```python
from build123d import *

# Parameters (mm, degrees)
F0_R     = 19.05
F1_DEPTH = 31.75
F2_R     = 5.5626
F3_DEPTH = 20.6502
F4_DEPTH = 57.151
F6_DEPTH = 4.7625


with BuildPart() as f1:
    # F0 (on Front) → F1 (new body, symmetric)
    with BuildSketch(Plane.XZ):
        with BuildLine():
            Line((50.8, 28.575), (0, 28.575))
            ThreePointArc((0, 28.575), (-15.0603473566, -24.2840804335), (25.5976683508, 12.7))
            Line((25.5976683508, 12.7), (50.8, 12.7))
            Line((50.8, 12.7), (50.8, 28.575))
        make_face()
        Circle(F0_R, mode=Mode.SUBTRACT)
    extrude(amount=F1_DEPTH, both=True)

    # F2 (on face) → F3 (join)
    with BuildSketch(Plane(origin=(0, 0, 12.7), x_dir=(1, 0, 0), z_dir=(0, 0, -1))):
        with BuildLine():
            Line((50.8, 24.6126), (50.8, 31.75))
            ThreePointArc((50.8, 31.75), (41.8197438789, 28.0302561211), (38.1, 19.05))
            Line((38.1, 19.05), (38.1, -19.05))
            ThreePointArc((38.1, -19.05), (41.8197438789, -28.0302561211), (50.8, -31.75))
            Line((50.8, -31.75), (50.8, -24.6126))
            ThreePointArc((50.8, -24.6126), (45.2374, -19.05), (50.8, -13.4874))
            Line((50.8, -13.4874), (50.8, 13.4874))
            ThreePointArc((50.8, 13.4874), (45.2374, 19.05), (50.8, 24.6126))
        make_face()
        with BuildLine():
            Line((90.4493554441, 11.0277214642), (57.0991554441, 30.0777214642))
            ThreePointArc((57.0991554441, 30.0777214642), (54.0586759125, 31.3248128824), (50.8, 31.75))
            Line((50.8, 31.75), (50.8, 24.6126))
            ThreePointArc((50.8, 24.6126), (54.733352181, 22.983352181), (56.3626, 19.05))
            ThreePointArc((56.3626, 19.05), (54.733352181, 15.116647819), (50.8, 13.4874))
            Line((50.8, 13.4874), (50.8, -13.4874))
            ThreePointArc((50.8, -13.4874), (54.733352181, -15.116647819), (56.3626, -19.05))
            ThreePointArc((56.3626, -19.05), (54.733352181, -22.983352181), (50.8, -24.6126))
            Line((50.8, -24.6126), (50.8, -31.75))
            ThreePointArc((50.8, -31.75), (54.0586759125, -31.3248128824), (57.0991554441, -30.0777214642))
            Line((57.0991554441, -30.0777214642), (90.4493554441, -11.0277214642))
            ThreePointArc((90.4493554441, -11.0277214642), (96.8502, 0), (90.4493554441, 11.0277214642))
        make_face()
        with Locations((84.1502, 0)):
            Circle(F2_R, mode=Mode.SUBTRACT)
    extrude(amount=-F3_DEPTH)

    # F4 (cut, through all): faces of the model
    f4_faces = [f1.faces().sort_by_distance(p)[0] for p in [
        (48.4391592362, 19.05, 28.575),
        (48.4391592362, -19.05, 28.575),
    ]]
    extrude(f4_faces, amount=-F4_DEPTH, mode=Mode.SUBTRACT)

    # F5 (on Front) → F6 (join, symmetric)
    with BuildSketch(Plane.XZ):
        with BuildLine():
            ThreePointArc((25.5976683508, 12.7), (27.6286795727, -7.2929205446), (15.9950252975, -23.6788891364))
            Line((15.9950252975, -23.6788891364), (69.85, 12.7))
            Line((69.85, 12.7), (25.5976683508, 12.7))
        make_face()
    extrude(amount=F6_DEPTH, both=True)


solid = f1.part
```
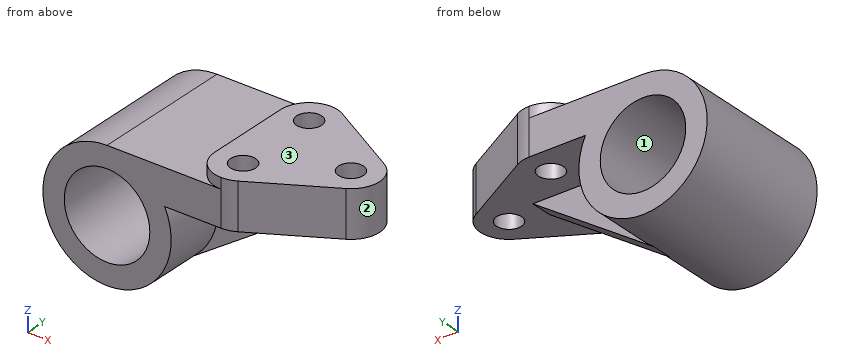
The listing builds one solid part. Answer for the finished solid, in the listing's coordinates (mm). Face numbers are marked on the shaded views. Give positions to 0.01 mm unless a question says otherwise; leave off trailing zeros. Loops run counter-clockwise (first coordinate to the right, second up) from the corner with the lowest first, then second, coordinate; pieces in that order, holes last. Notation, with made-up numbers: (-37.75, 70.5) - (18.25, 70.5) arc R32 ccw to (18.25, 101.5) - close; hole circle Ø1 at (7, 61). An arc over 180 degrees is marked (long way). Answer as CSV lines item,"result". Start each with the question number.
Item 1: Each of these flat-tipped pins is pushed along its axis until it touches: pin 1 (4 mm diameter, centred on y = 2, z = 32, fed in from -X); pin 2 (12 mm diameter, centred on x = 32.5, y = -22, fed in from -Z); pin 3 (18 mm diameter, centred on x = 50.8, y = 19.05, fed in from -Z); pin 4 (10 mm diameter, centred on x = 84.15, y = 0, fed in from -Z). Where does it stop, or does it pass through?
Item 2: A cutting plane is placed at C-C on z = 2. Determine the outline of the cut face in (x, y), then the cut area to 3 significant figures.
Item 3: A cutting plane is placed at A-A on y = 17.5. Determine the outline of the cut face in (x, z) (3 decimals), then the cut area to 3 significant figures.
Item 4: Find the intervals of material crossed by line 1 (Y direction, x = 50.8, z = 28.25); line 2 (Y direction, x = 54.5, z = 28.5); line 3 (Z direction, x = 0, y = 17) (3 decimals), in increasing order. Write a range as from..to.
Item 5: A cutting plane is placed at D-D on y = 27. Determine the outline of the cut face in (x, z) (3 decimals), then the cut area to 3 significant figures.
Item 6: The mould has two halves that part along Z. Classify the marked faces 1, 2 and 3: +Z half, -Z half, draft (parallel to the pull), parting line (faces both ways), or undercut.
Item 7: A cutting plane is placed at B-B on x = -1.5. Determine the outline of the cut face in (y, z).
Found:
1,pin 1,"stops at x = 38.1"
1,pin 2,"stops at z = -10.69"
1,pin 3,"stops at z = 12.7"
1,pin 4,"passes through"
2,outline,"(-28.5, -31.75) - (-18.94, -31.75) - (-18.94, 31.75) - (-28.5, 31.75) - close; (18.94, -31.75) - (28.5, -31.75) - (28.5, -4.76) - (54.01, -4.76) - (54.01, 4.76) - (28.5, 4.76) - (28.5, 31.75) - (18.94, 31.75) - close"
2,area,"1,460 mm^2"
3,outline,"(0, 28.575) arc R28.575 ccw (long way) to (25.598, 12.7) - (45.458, 12.7) - (45.458, 33.35) - (38.1, 33.35) - (38.1, 28.575) - close; (56.142, 12.7) - (79.119, 12.7) - (79.119, 33.35) - (56.142, 33.35) - close; hole circle Ø38.1 at (0, 0)"
3,area,"2,370 mm^2"
4,line 1,"y = -31.75..-24.61, -13.49..13.49, 24.61..31.75"
4,line 2,"y = -31.2..-23.2, -14.9..14.9, 23.2..31.2"
4,line 3,"z = -28.575..-19.05, 19.05..28.575"
5,outline,"(0, 28.575) arc R28.575 ccw (long way) to (25.598, 12.7) - (62.487, 12.7) - (62.487, 33.35) - (40.896, 33.35) - (40.896, 28.575) - close; hole circle Ø38.1 at (0, 0)"
5,area,"2,230 mm^2"
6,face 1,"undercut"
6,face 2,"draft"
6,face 3,"+Z half"
7,outline,"(-31.75, -28.54) - (31.75, -28.54) - (31.75, -18.99) - (-31.75, -18.99) - close; (-31.75, 18.99) - (31.75, 18.99) - (31.75, 28.54) - (-31.75, 28.54) - close"
